For this review, take the finished solid that the model builds, in its own axes (mm). A direction names the side the tool comes from. Round coordinates to 2 decimals unless told otherwise and drop trailing zeros. Loops run counter-clockwise (first coordinate to the right, second up) from the corner with the lowest first, then second, coordinate; pieces in that order, holes last.
1. Consider section D-D on y = 13.2. State the section outline as (x, z) points, then the cut area to 3 significant figures.
2. Draft analysis for pull direction Z (two halves, no side actions). For faces 1 (the cylindrical face through (101.279, 40.831, -66.453)), 2 (the flat face through (70, 44, -8.7)), 3 (the flat face through (99.8, 34, -50)), 4 (the flat face through (94.8, 45, -51)), state which applies: released by +Z, released by -Z, zero draft, split by the parting line, or undercut.
3. Clearance check with flat-ended pins moving along their axes: pin 1 Ø1.5 at (y, z) = (61, -69.5) entering from +X; pin 2 Ø1.2 at (x, z) = (81, -14.5) entering from +Y; pin 3 Ø18 at (y, z) = (43, -38) entering from -X. State where each tip first meets the part, or that it passes through.
4. To check wall thickness, follow line 1 along Z through (x, y) = (95, 55); line 2 along X through (y, z) = (32.5, -49.5); line 3 along X through (y, z) = (6, -21). State the ranges of each line that lie inside material, in increasing order.
5. Consider section C-C on z = -31. State the section outline as (x, y) points, then the cut area to 3 significant figures.
6. Consider section A-A on x = 70.5. State the section outline as (y, z) points.
7. Consider section B-B on y = 60.3. State how many separate pieces and enclosed holes the cut face has, then the cut area to 3 significant figures.
8. Tool access review of faces 5 (the flat face through (63, 5, -12)), 6 (the flat face through (98.856, 68.326, -49.698)), 7 (the flat face through (83, 0.2, -10)), 8 (the cylindrical face through (31.85, 61.33, -10.18)), 9 (the flat face through (81, 3.664, -14)): name each direction out of +Z, -Z, +X, -X, +Y, -Y from which nothing blocks a thin tool from reaching the whole face with its end or side.
from build123d import *

# Parameters (mm, degrees)
SKETCH040_R     = 1.7
PAD021_DEPTH    = 3
PAD022_DEPTH    = 3
SKETCH041_R     = 2.2
POCKET013_DEPTH = 26.619333
PAD020_DEPTH    = 5
PAD023_DEPTH    = 4
POCKET015_DEPTH = 31.8
POCKET014_DEPTH = 80.219333


with BuildPart() as part:
    # Sketch040 (on Face4 of Binder004) → Pad021 (new body)
    with BuildSketch(Plane(origin=(0, 0, -8.7), x_dir=(1, 0, 0), z_dir=(0, 0, -1))):
        Polygon((63, -0.2), (63, -10.2), (14.581667, -73.3), (126.418333, -73.3), (102.8, -42.519989), (102.8, -0.2), align=None)
        with Locations((70.5, -13.2)):
            Circle(SKETCH040_R, mode=Mode.SUBTRACT)
        with Locations((107.8, -60.3)):
            Circle(SKETCH040_R, mode=Mode.SUBTRACT)
        with Locations((33.2, -60.3)):
            Circle(SKETCH040_R, mode=Mode.SUBTRACT)
    extrude(amount=PAD021_DEPTH)

    # Sketch042 (on Face6 of Pad021) → Pad022 (join)
    with BuildSketch(Plane.YZ.offset(102.8)):
        Polygon((0.2, -11.7), (48.475, -95.314753), (83.116016, -75.314753), (53.116016, -23.353229), (73.3, -11.7), align=None)
    extrude(amount=-PAD022_DEPTH)

    # Sketch041 (on Face14 of Pad022) → Pocket013 (cut, through all)
    with BuildSketch(Plane(origin=(99.8, 0, 0), x_dir=(0, -1, 0), z_dir=(-1, 0, 0))):
        with Locations((-51.846002, -81.821499)):
            Circle(SKETCH041_R)
        with Locations((-41.846002, -64.500991)):
            Circle(SKETCH041_R)
        with Locations((-64.16651, -63.161245)):
            Circle(SKETCH041_R)
    extrude(amount=-POCKET013_DEPTH, mode=Mode.SUBTRACT)

    # Sketch043 (on Face14 of Pocket013) → Pad020 (join)
    with BuildSketch(Plane(origin=(99.8, 0, 0), x_dir=(0, -1, 0), z_dir=(-1, 0, 0))):
        Polygon((-0.2, -11.7), (-48.475, -95.314753), (-51.073076, -93.814753), (-3.664102, -11.7), align=None)
        Polygon((-42.92392, -11.7), (-80.51794, -76.814753), (-83.116016, -75.314753), (-53.116016, -23.353229), (-73.3, -11.7), align=None)
        Polygon((-21.56196, -11.7), (-64.49647, -86.064753), (-67.094546, -84.564753), (-25.026062, -11.7), align=None)
    extrude(amount=PAD020_DEPTH)

    # Sketch038 (on Face5 of Pad020) → Pad023 (join)
    with BuildSketch(Plane(origin=(0, 0, -11.7), x_dir=(1, 0, 0), z_dir=(0, 0, -1))):
        Polygon((94.8, -3.664102), (66, -3.664102), (66, -11.218363), (20.665065, -70.3), (57.401987, -70.3), (94.8, -21.56196), (94.8, -25.026062), (60.060085, -70.3), (94.8, -70.3), (94.8, -73.3), (14.581667, -73.3), (63, -10.2), (63, -0.2), (94.8, -0.2), align=None)
    extrude(amount=PAD023_DEPTH)

    # Sketch044 (on Face16 of Pad023) → Pocket015 (cut)
    with BuildSketch(Plane.YZ.offset(94.8)):
        Polygon((2.509401, -15.7), (0.2, -15.7), (0.2, -11.7), align=None)
        Polygon((23.871361, -15.7), (21.56196, -11.7), (21.56196, -15.7), align=None)
    extrude(amount=-POCKET015_DEPTH, mode=Mode.SUBTRACT)

    # Sketch039 (on Face30 of Pocket015) → Pocket014 (cut, through all)
    with BuildSketch(Plane.YZ.offset(94.8)):
        Polygon((73.3, -11.7), (73.3, -15.7), (66.371797, -15.7), align=None)
    extrude(amount=-POCKET014_DEPTH, mode=Mode.SUBTRACT)


solid = part.part
Resolved:
1. outline: (60.7, -15.7) - (64.48, -15.7) - (64.48, -11.7) - (68.8, -11.7) - (68.8, -8.7) - (60.7, -8.7) - close; (72.2, -11.7) - (99.8, -11.7) - (99.8, -28.22) - (94.8, -28.22) - (94.8, -34.22) - (102.8, -34.22) - (102.8, -8.7) - (72.2, -8.7) - close
1. area: 229 mm2
2. face 1: undercut
2. face 2: released by +Z
2. face 3: undercut
2. face 4: zero draft
3. pin 1: stops at x = 102.8
3. pin 2: stops at y = 43.79
3. pin 3: stops at x = 94.8
4. line 1: z = -69.62 to -63.62, -32.62 to -26.62, -22.27 to -8.7
4. line 2: x = 99.8 to 102.8
4. line 3: x = 94.8 to 102.8
5. outline: (94.8, 11.34) - (102.8, 11.34) - (102.8, 57.53) - (94.8, 57.53) - (94.8, 54.07) - (99.8, 54.07) - (99.8, 36.17) - (94.8, 36.17) - (94.8, 32.7) - (99.8, 32.7) - (99.8, 14.81) - (94.8, 14.81) - close
5. area: 191 mm2
6. outline: (0.2, -11.7) - (2.51, -15.7) - (3.66, -15.7) - (3.66, -11.7) - (11.5, -11.7) - (11.5, -8.7) - (0.2, -8.7) - close; (14.9, -11.7) - (53.23, -11.7) - (53.23, -15.7) - (56.69, -15.7) - (56.69, -11.7) - (70.3, -11.7) - (70.3, -13.43) - (73.3, -11.7) - (73.3, -8.7) - (14.9, -8.7) - close
7. separate pieces: 4
7. enclosed holes: 0
7. area: 559 mm2
8. face 5: +Z, -Z, -X, -Y
8. face 6: +X, -X, +Y
8. face 7: +Z, -Z, +X, -X, -Y
8. face 8: +Z, -Z
8. face 9: -Z
